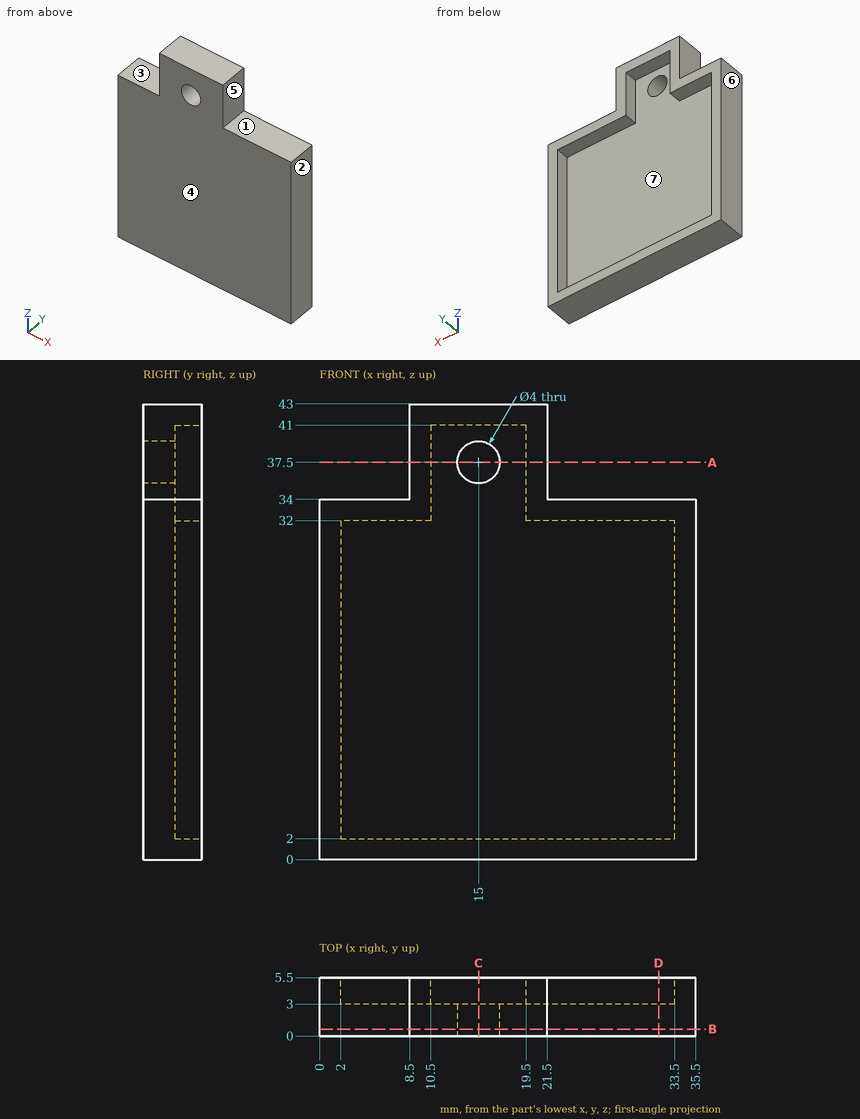
Here's the drawing with two shaded views (mm, measured from the low corner). I have some questions. A direction names the side the tool comes from. Coordinates: 2 decimals unless noted, no trailing zeros. Loops run counter-clockwise (first coordinate to the right, second up) from the corner with the lowest first, then second, coordinate; pieces in that order, holes last. Notation, with made-up numbers: (14.5, 24.25) -> (73.5, 24.25) arc R24 ccw to (73.5, 54.25) -> close; hole circle Ø10 at (-35, -20.75). An arc over 180 degrees is marked (long way). Answer as a JSON object with one key per item and string values.
1) For the marked faces 1, 2 and 3, which set-ups out of +Z, -Z, +X, -X, +Y, -Y let a thin tool reach every point of the face, with its end or its side?
Results:
{"face 1": "+Z, +X, +Y, -Y", "face 2": "+Z, -Z, +X, +Y, -Y", "face 3": "+Z, -X, +Y, -Y"}
2) For P1, Ø1, axis at x = 30.5, z = 35, coming from the -Y side; P2, Ø0.8, axis at y = 3.5, z = 34.5, coming from the -X side; P3, Ø1.6, axis at x = 31.5, y = 4, coming from the +Z side; P4, Ø3, axis at y = 2, z = 38.5, coming from the +X side, each with a flat end and sliding along its axis, tell me the tip position at first contact or that it passes through.
Results:
{"P1": "passes through", "P2": "stops at x = 8.5", "P3": "stops at z = 34", "P4": "stops at x = 21.5"}
3) If I drill on line 1 (Z direction, x = 15, y = 0.65); line 2 (X direction, y = 0.7, z = 37.5); line 3 (X direction, y = 4.1, z = 40), over which ranges is the centre line in solid material (lowest first)?
Results:
{"line 1": "z = 0 to 35.5, 39.5 to 43", "line 2": "x = 8.5 to 13, 17 to 21.5", "line 3": "x = 8.5 to 10.5, 19.5 to 21.5"}
4) Imagine slicing it at A-A (z = 37.5). Please give me the cut outline in (x, y), then the cut area to 3 significant figures.
Results:
{"outline": "(8.5, 0) -> (13, 0) -> (13, 3) -> (10.5, 3) -> (10.5, 5.5) -> (8.5, 5.5) -> close; (17, 0) -> (21.5, 0) -> (21.5, 5.5) -> (19.5, 5.5) -> (19.5, 3) -> (17, 3) -> close", "area": "37.0 mm^2"}
5) Imagine slicing it at B-B (y = 0.65). Please give me the cut outline in (x, z).
Results:
{"outline": "(0, 0) -> (35.5, 0) -> (35.5, 34) -> (21.5, 34) -> (21.5, 43) -> (8.5, 43) -> (8.5, 34) -> (0, 34) -> close; hole circle Ø4 at (15, 37.5)"}
6) Imagine slicing it at C-C (x = 15). Please give me the cut outline in (y, z).
Results:
{"outline": "(0, 0) -> (5.5, 0) -> (5.5, 2) -> (3, 2) -> (3, 35.5) -> (0, 35.5) -> close; (0, 39.5) -> (3, 39.5) -> (3, 41) -> (5.5, 41) -> (5.5, 43) -> (0, 43) -> close"}
7) Imagine slicing it at D-D (x = 32). Please give me the cut outline in (y, z), then the cut area to 3 significant figures.
Results:
{"outline": "(0, 0) -> (5.5, 0) -> (5.5, 2) -> (3, 2) -> (3, 32) -> (5.5, 32) -> (5.5, 34) -> (0, 34) -> close", "area": "112 mm^2"}
8) Thinking about a two-plate mould opening in X: for the marked faces 4, 5, 6 and 7, which applies, pulls with the +X half, pulls with the -X half, needs draft (parallel to the pull), parting line crosses it, or undercut?
Results:
{"face 4": "needs draft", "face 5": "pulls with the +X half", "face 6": "pulls with the -X half", "face 7": "undercut"}
